Can you work these out from the model? Positions are in its coordinate system, mm. A direction names the side the tool comes from. Coordinates: 2 decimals unless noted, no trailing zeros. Loops run counter-clockwise (first coordinate to the right, second up) from the corner with the lowest first, then second, coordinate; pieces in that order, holes last. Notation, with made-up numbers: M 38.5,-28 L 78.5,-28 A22 ccw 78.5,-1 Z; hole C 18.5,34.5 d1. An arc over 180 degrees is marked long. Answer as a JSON object with one key per item and string values. Group by question number.
Item 1: Suppose I cut it at D-D (y = 47). Write out the boundary of the cut face in (x, z).
Item 2: If I drill on line 1 (X direction, y = 69, z = 5.25); line 2 (X direction, y = 102.5, z = 3); line 3 (X direction, y = 99, z = 15.75), over which ranges is the centre line in solid material (lowest first)?
Item 3: Suppose I cut it at C-C (x = -28.5). Write out the boundary of the cut face in (y, z).
Item 4: We'd pull the mould along X, two halves only. Please class faces 3 (the flat face through (-24.3, 66.1, 0)), 4 (the flat face through (-25.6, 55, 10)), 5 (the cylindrical face through (-34.25, 87.66, 9.86)), 6 (the cylindrical face through (-1.487, 168.974, 9.86)): +X half, -X half, draft (parallel to the pull), parting line (faces both ways), or undercut.
Item 5: Suppose I cut it at A-A (y = 116). Write out the boundary of the cut face in (x, z).
Item 6: Which directions (+Z, -Z, +X, -X, +Y, -Y) give clear straight access to the entire face, cutting with the end or side of a thin tool? Please do faces 1 (the cylindrical face through (-3.025, 155.315, 9.86)), 2 (the flat face through (-23, 0, 10)).
Item 7: Suppose I cut it at B-B (z = 15). Count the separate pieces of the cut face and the enclosed holes in it, then the cut area to 3 significant figures.
Item 8: I'm going to push flat-ended pins straight in: pin 1 Ø4 at (x, z) = (-16.5, 7.5) entering from +Y; pin 2 Ø2 at (x, z) = (-19.5, 7.5) entering from +Y; pin 3 Ø1.5 at (x, y) = (-31, 70.5) entering from -Z; pin 4 Ø10 at (y, z) = (48, 12.5) entering from -X. Where does each tip first touch, or does it pass through?
```python
from build123d import *

# Parameters (mm, degrees)
BOSS_EXTRUDE4_DEPTH  = 20
SKETCH12_R           = 1.65
CUT_EXTRUDE1_DEPTH   = 177.068006068
SKETCH14_W           = 1.5
SKETCH14_H           = 148.56444562
BOSS_EXTRUDE5_DEPTH  = 20
CUT_EXTRUDE2_START   = -20
CUT_EXTRUDE2_DEPTH   = 20
CUT_EXTRUDE3_START   = -30
CUT_EXTRUDE3_DEPTH   = 30
LPATTERN2_COUNT      = 5
LPATTERN2_PITCH      = 8
LPATTERN2_COUNT_DIR2 = 5
LPATTERN2_PITCH_DIR2 = 8
CUT_EXTRUDE4_START   = -30
CUT_EXTRUDE4_DEPTH   = 30


with BuildPart() as part:
    # Sketch5 → Boss-Extrude4 (new body)
    with BuildSketch(Plane.XY):
        with BuildLine():
            Line((0, 0), (0, 167.041245738))
            ThreePointArc((0, 167.041245738), (-1.523254023, 168.9835931), (-3.772713274, 167.967252028))
            ThreePointArc((-3.772713274, 167.967252028), (-34.542452011, 86.476422979), (-45, 0))
            Line((-45, 0), (0, 0))
        make_face()
        with BuildLine():
            Line((-1.6, 10), (-39.860221142, 10))
            ThreePointArc((-39.860221142, 10), (-30.000299364, 83.996114978), (-5, 154.335493145))
            ThreePointArc((-5, 154.335493145), (-2.992115624, 155.307611869), (-1.6, 153.56444562))
            Line((-1.6, 153.56444562), (-1.6, 10))
        make_face(mode=Mode.SUBTRACT)
    extrude(amount=BOSS_EXTRUDE4_DEPTH)

    # Sketch12 → Cut-Extrude1 (cut, through all)
    with BuildSketch(Plane.XY.offset(20)):
        with Locations((-40, 5)):
            Circle(SKETCH12_R)
        with Locations((-22.5, 5)):
            Circle(SKETCH12_R)
        with Locations((-5, 5)):
            Circle(SKETCH12_R)
    extrude(amount=-CUT_EXTRUDE1_DEPTH, mode=Mode.SUBTRACT)

    # Sketch14 → Boss-Extrude5 (add)
    with BuildSketch(Plane.XY.offset(20)):
        with Locations((-0.85, 84.28222281)):
            Rectangle(SKETCH14_W, SKETCH14_H)
    boss_extrude5 = extrude(amount=-BOSS_EXTRUDE5_DEPTH)

    # Sketch17 → Cut-Extrude2 (cut)
    with BuildSketch(Plane.XY.offset(20).offset(CUT_EXTRUDE2_START)):
        Polygon((-120.638203698, 868.825955305), (-109.129206393, -31.174044695), (790.870793607, -19.66504739), (784.13367644, 507.175413991), align=None)
        with BuildLine():
            Line((-45, 0), (0, 0))
            Line((0, 0), (0, 167.041245738))
            ThreePointArc((0, 167.041245738), (-1.523254023, 168.9835931), (-3.772713274, 167.967252028))
            ThreePointArc((-3.772713274, 167.967252028), (-34.542452011, 86.476422979), (-45, 0))
        make_face(mode=Mode.SUBTRACT)
    extrude(amount=CUT_EXTRUDE2_DEPTH, mode=Mode.SUBTRACT)

    # Sketch18 → Cut-Extrude3 (cut)
    with BuildSketch(Plane.XY.offset(20).offset(CUT_EXTRUDE3_START)):
        Polygon((10.567687301, -7.152622061), (26.572035637, 318.782087337), (-234.729728554, 306.471050155), (-205.798791176, -46.855716973), align=None)
        with BuildLine():
            Line((-45, 0), (0, 0))
            Line((0, 0), (0, 167.041245738))
            ThreePointArc((0, 167.041245738), (-1.523254023, 168.9835931), (-3.772713274, 167.967252028))
            ThreePointArc((-3.772713274, 167.967252028), (-34.542452011, 86.476422979), (-45, 0))
        make_face(mode=Mode.SUBTRACT)
    extrude(amount=CUT_EXTRUDE3_DEPTH, mode=Mode.SUBTRACT)

    # LPattern2: Boss-Extrude5 5 × 5, 10 skipped
    with Locations(*[Vector(-1, 0, 0) * (i * LPATTERN2_PITCH) + Vector(-1, 0, 0) * (j * LPATTERN2_PITCH_DIR2) for i in range(LPATTERN2_COUNT) for j in range(LPATTERN2_COUNT_DIR2) if (i, j) not in ((0, 0), (1, 4), (2, 3), (2, 4), (3, 2), (3, 3), (3, 4), (4, 1), (4, 2), (4, 3), (4, 4))]):
        add(boss_extrude5)

    # Sketch19 → Cut-Extrude4 (cut)
    with BuildSketch(Plane.XY.offset(20).offset(CUT_EXTRUDE4_START)):
        Polygon((-113.909990018, -19.131609845), (183.246695872, -29.17634289), (134.697152825, 220.267861041), (-171.248674479, 235.334960607), align=None)
        with BuildLine():
            Line((-45, 0), (0, 0))
            Line((0, 0), (0, 167.041245738))
            ThreePointArc((0, 167.041245738), (-1.523254023, 168.9835931), (-3.772713274, 167.967252028))
            ThreePointArc((-3.772713274, 167.967252028), (-34.542452011, 86.476422979), (-45, 0))
        make_face(mode=Mode.SUBTRACT)
    extrude(amount=CUT_EXTRUDE4_DEPTH, mode=Mode.SUBTRACT)


solid = part.part
```
From the geometry:
{
 "1": {"outline": "M -41.94,0 L -36.9,0 L -36.9,20 L -41.94,20 Z; M -33.6,0 L -32.1,0 L -32.1,20 L -33.6,20 Z; M -25.6,0 L -24.1,0 L -24.1,20 L -25.6,20 Z; M -17.6,0 L -16.1,0 L -16.1,20 L -17.6,20 Z; M -9.6,0 L -8.1,0 L -8.1,20 L -9.6,20 Z; M -1.6,0 L 0,0 L 0,20 L -1.6,20 Z"},
 "2": {"line 1": "-38.38 to -32.1, -25.6 to -24.1, -17.6 to -16.1, -9.6 to -8.1, -1.6 to 0", "line 2": "-30.22 to -24.1, -17.6 to -16.1, -9.6 to -8.1, -1.6 to 0", "line 3": "-31.23 to -26.03, -25.6 to -24.1, -17.6 to -16.1, -9.6 to -8.1, -1.6 to 0"},
 "3": {"outline": "M 0,0 L 10,0 L 10,20 L 0,20 Z; M 89.98,0 L 108.16,0 L 108.16,20 L 89.98,20 Z"},
 "4": {"face 3": "draft", "face 4": "undercut", "face 5": "-X half", "face 6": "parting line"},
 "5": {"outline": "M -25.95,0 L -20.67,0 L -20.67,20 L -25.95,20 Z; M -17.6,0 L -16.1,0 L -16.1,20 L -17.6,20 Z; M -9.6,0 L -8.1,0 L -8.1,20 L -9.6,20 Z; M -1.6,0 L 0,0 L 0,20 L -1.6,20 Z"},
 "6": {"face 1": "+Z, -Z", "face 2": "+Z, -Z, +X, -X, -Y"},
 "7": {"separate pieces": "1", "enclosed holes": "8", "area": "2,110 mm2"},
 "8": {"pin 1": "y = 145.6", "pin 2": "y = 136.11", "pin 3": "through", "pin 4": "x = -42.44"}
}
